from build123d import *

# Parameters (mm, degrees)
SKETCH1_R           = 9.525
BOSS_EXTRUDE2_DEPTH = 101.6
SKETCH3_R           = 4.7625
BOSS_EXTRUDE3_DEPTH = 12.7
SKETCH14_R          = 5.7546875
CUT_EXTRUDE4_DEPTH  = 25.4
SKETCH17_R          = 1.905
CUT_EXTRUDE5_DEPTH  = 89.9


with BuildPart() as part:
    # Sketch1 → Boss-Extrude2 (new body)
    with BuildSketch(Plane(origin=(0, 0, 0), x_dir=(1, 0, 0), z_dir=(0, 1, 0))):
        Circle(SKETCH1_R)
    extrude(amount=BOSS_EXTRUDE2_DEPTH)

    # Sketch3 → Boss-Extrude3 (add)
    with BuildSketch(Plane(origin=(0, 101.6, 0), x_dir=(1, 0, 0), z_dir=(0, 1, 0))):
        Circle(SKETCH3_R)
    extrude(amount=BOSS_EXTRUDE3_DEPTH)

    # Sketch14 → Cut-Extrude4 (cut)
    with BuildSketch(Plane.XZ):
        Circle(SKETCH14_R)
    extrude(amount=-CUT_EXTRUDE4_DEPTH, mode=Mode.SUBTRACT)

    # Sketch17 → Cut-Extrude5 (cut, through all)
    with BuildSketch(Plane.XZ.offset(-25.4)):
        Circle(SKETCH17_R)
    extrude(amount=-CUT_EXTRUDE5_DEPTH, mode=Mode.SUBTRACT)


solid = part.part
Geometry: final body of the model. Coordinates: model frame, mm. A direction names the side the tool comes from. Give positions to 0.01 mm unless a question says otherwise; leave off trailing zeros. Loops run counter-clockwise (first coordinate to the right, second up) from the corner with the lowest first, then second, coordinate; pieces in that order, holes last. Notation, with made-up numbers: (-14, 77) - (11, 77) arc R30 ccw to (11, 100) - close; hole circle Ø1 at (-24, -10.75). An arc over 180 degrees is marked (long way). Answer as CSV lines item,"result". Start each with the question number.
1. Pin query (flat end, axial travel): P1, Ø3.5, axis at x = 2.5, z = -2.5, coming from the -Y side; P2, Ø10, axis at y = 99.5, z = 6, coming from the -X side; P3, Ø3, axis at y = 94, z = -2.5, coming from the +X side; P4, Ø3.5, axis at x = 0, z = 0, coming from the -Y side. Return the tip coordinate at first contact, or that it passes through.
2. Section B-B, the plane z = 0. Return loops of the section in (x, y) (1 decimal).
3. Section C-C, the plane y = 28. Return loops of the section in (x, z) (3 decimals), plus the area to 3 significant figures.
4. Ray query, L1, parallel to Z at x = 0, y = 7.5 (3 decimals); L2, parallel to Z at x = 0.25, y = 69; L3, parallel to Y at x = -3.75, z = -1.5. Return the intervals inside material, ascending.
5. Section A-A, the plane x = 0. Return loops of the section in (y, z) (1 decimal), plus the area to 3 significant figures.
6. Section D-D, the plane x = -7.75. Return loops of the section in (y, z), plus the area to 3 significant figures.
7. Reachability of faces 4 (the face through (-3.78, 107.86, 2.9)), 5 (the face through (-4.57, 12.52, -3.5)), 6 (the face through (-0.41, 69.23, -1.86)) from +Z, -Z, +X, -X, +Y, -Y: full face, straight path, thin tool, end or side. Return the list, or none.
8. Draft query along X for faces 1 (the face through (-7.559, 50.089, 5.796)), 2 (the face through (2.5, 25.4, 0.1)), 3 (the face through (0, 0, 6)). Return one class per face: released by +X, released by -X, zero draft, split by the parting line, or undercut.
Answers:
1,P1,"stops at y = 25.4"
1,P2,"stops at x = -9.47"
1,P3,"stops at x = 9.47"
1,P4,"passes through"
2,outline,"(-9.5, 0) - (-5.8, 0) - (-5.8, 25.4) - (-1.9, 25.4) - (-1.9, 114.3) - (-4.8, 114.3) - (-4.8, 101.6) - (-9.5, 101.6) - close; (1.9, 25.4) - (5.8, 25.4) - (5.8, 0) - (9.5, 0) - (9.5, 101.6) - (4.8, 101.6) - (4.8, 114.3) - (1.9, 114.3) - close"
3,outline,"circle Ø19.05 at (0, 0); hole circle Ø3.81 at (0, 0)"
3,area,"274 mm2"
4,L1,"z = -9.525 to -5.755, 5.755 to 9.525"
4,L2,"z = -9.52 to -1.89, 1.89 to 9.52"
4,L3,"y = 25.4 to 114.3"
5,outline,"(0, -9.5) - (101.6, -9.5) - (101.6, -4.8) - (114.3, -4.8) - (114.3, -1.9) - (25.4, -1.9) - (25.4, -5.8) - (0, -5.8) - close; (0, 5.8) - (25.4, 5.8) - (25.4, 1.9) - (114.3, 1.9) - (114.3, 4.8) - (101.6, 4.8) - (101.6, 9.5) - (0, 9.5) - close"
5,area,"1,430 mm2"
6,outline,"(0, -5.54) - (101.6, -5.54) - (101.6, 5.54) - (0, 5.54) - close"
6,area,"1,130 mm2"
7,face 4,"+Y"
7,face 5,"-Y"
7,face 6,"+Y, -Y"
8,face 1,"split by the parting line"
8,face 2,"undercut"
8,face 3,"zero draft"
